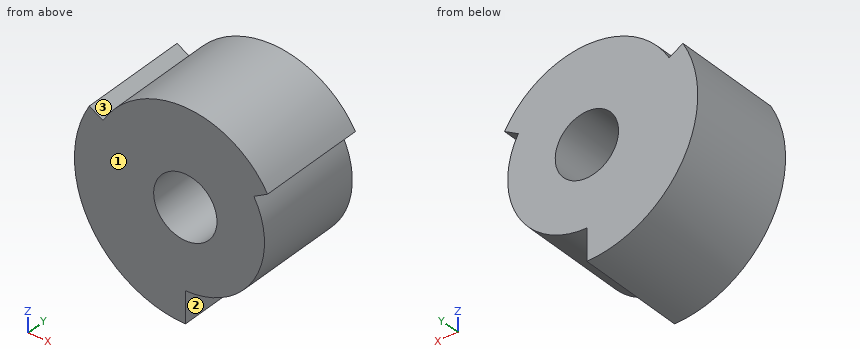
```python
from build123d import *

# Parameters (mm, degrees)
SKETCH1_R           = 10
BOSS_EXTRUDE1_DEPTH = 35


with BuildPart() as part:
    # Sketch1 → Boss-Extrude1 (new body)
    with BuildSketch(Plane(origin=(0, 0, 0), x_dir=(1, 0, 0), z_dir=(0, 1, 0))):
        with BuildLine():
            Line((0, 25), (0, 30))
            Line((0, 30), (0, 35))
            ThreePointArc((0, 35), (-30.310889132, 17.5), (-30.310889132, -17.5))
            Line((-30.310889132, -17.5), (-25.980762114, -15))
            ThreePointArc((-25.980762114, -15), (0, -30), (25.980762114, -15))
            Line((25.980762114, -15), (21.650635095, -12.5))
            ThreePointArc((21.650635095, -12.5), (21.650635095, 12.5), (0, 25))
        make_face()
        with Locations(Location((0, 0, 0), (0, 0, 270))):
            Circle(SKETCH1_R, mode=Mode.SUBTRACT)
    extrude(amount=BOSS_EXTRUDE1_DEPTH)


solid = part.part
```
Part model, mm, in its own coordinate system. Face numbers are marked on the shaded views. Round coordinates to 2 decimals unless told otherwise and drop trailing zeros. Write each loop counter-clockwise with the first axis right and the second up, starting at its lowest first coordinate (ties: lowest second). Pieces come first, ordered by that corner, then holes.
Item 1: Probe L1, parallel to X at y = 15, z = 0; L2, parallel to Z at x = -0.5, y = 28.5; L3, parallel to X at y = 30.5, z = 4. List the from-to ranges inside material, lowest first.
Results:
L1: x = -35 to -10, 10 to 25
L2: z = -35 to -9.99, 9.99 to 30
L3: x = -34.77 to -9.17, 9.17 to 24.68
Item 2: Drop flat-ended pins along their axis: pin 1 Ø1 at (x, y) = (15, 11.5) entering from -Z; pin 2 Ø4 at (x, y) = (-10.5, 8) entering from +Z; pin 3 Ø1.5 at (y, z) = (24, 7.5) entering from +X; pin 4 Ø16 at (x, z) = (0, 0) entering from +Y. Give the stop position or say it passes through.
Results:
pin 1: stops at z = -20.37
pin 2: stops at z = 28.77
pin 3: stops at x = 24.07
pin 4: passes through
Item 3: Two-plate mould, pull along X, no slides. Class the marked faces 1, 2 and 3: +X half, -X half, draft (parallel to the pull), parting line (faces both ways), or undercut.
Results:
face 1: draft
face 2: +X half
face 3: undercut
Item 4: Cut at D-D, the plane z = -23. Give the cut face in (x, y), plus the area to 3 significant figures.
Results:
outline: (-26.38, 0) - (9.8, 0) - (9.8, 35) - (-26.38, 35) - close
area: 1,270 mm2
Item 5: Cut at C-C, the plane y = 28. Give the cut face in (x, z), plus the area to 3 significant figures.
Results:
outline: (-30.31, 17.5) arc R35 ccw to (0, -35) - (0, -25) arc R25 ccw to (21.65, 12.5) - (25.98, 15) arc R30 ccw to (-25.98, 15) - close; hole circle Ø20 at (0, 0)
area: 2,570 mm2
Item 6: Cut at B-B, the plane x = 3.5. Give the cut face in (y, z).
Results:
outline: (0, -24.75) - (35, -24.75) - (35, -9.37) - (0, -9.37) - close; (0, 9.37) - (35, 9.37) - (35, 29.8) - (0, 29.8) - close
Item 7: Cut at A-A, the plane z = 0. Give the cut face in (x, y), plus the area to 3 significant figures.
Results:
outline: (-35, 0) - (-10, 0) - (-10, 35) - (-35, 35) - close; (10, 0) - (25, 0) - (25, 35) - (10, 35) - close
area: 1,400 mm2
